Could you check a few things on this drawing? It's one solid part, dimensions in mm from its lowest x, y, z. A direction names the side the tool comes from. Give positions to 0.01 mm unless a question says otherwise; leave off trailing zeros. Loops run counter-clockwise (first coordinate to the right, second up) from the corner with the lowest first, then second, coordinate; pieces in that order, holes last.
Q1. Suppose I cut it at A-A (x = 25). List the corners of the cut face in (y, z) for me.
Q2. Thinking about a two-plate mould opening in Z: for the marked faces 1, 2 and 3, which applies, pulls with the +Z half, pulls with the -Z half, needs draft (parallel to the pull), parting line crosses it, or undercut?
Q3. I'm going to push a flat-ended pin straight in: P1, Ø6, axis at y = 23, z = 22, coming from the +X side. Where does the tip first touch, or does it pass through?
Q4. Suppose I cut it at C-C (y = 30). List the corners of the cut face in (x, z) for me.
Q5. Suppose I cut it at B-B (z = 20). List the corners of the cut face in (x, y) for me.
Q6. I need wall thicknesses on probe 1 along X at (y, z) = (11, 35); probe 2 along Z at (x, y) = (7, 14) (1 decimal); probe 3 along Z at (x, y) = (33, 12.5). Which ranges of each line are inside material? Lowest first, please.
Q7. Suppose I cut it at D-D (z = 24.5). List the corners of the cut face in (x, y) for me, and give its area (3 significant figures).
Q8. For the marked faces 4 and 5, which set-ups out of +Z, -Z, +X, -X, +Y, -Y let a thin tool reach every point of the face, with its end or its side?
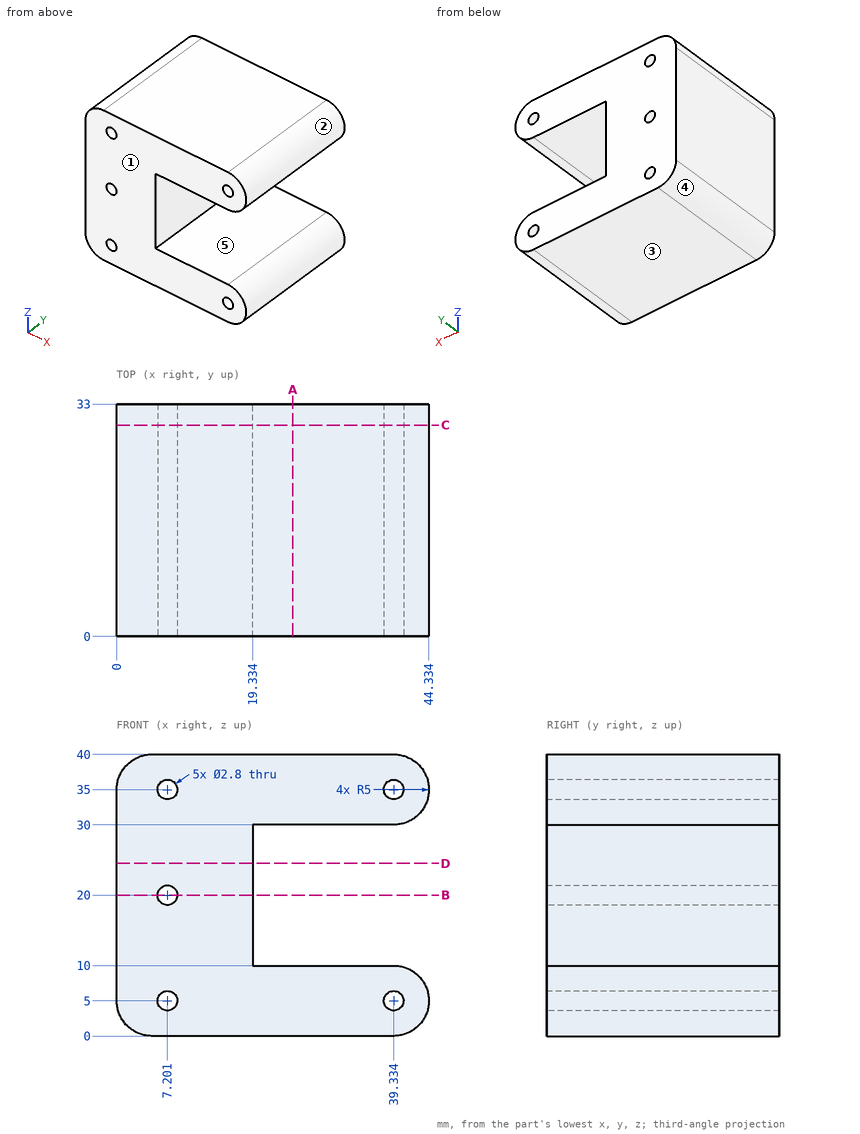
Solutions:
1. outline: (0, 0) - (33, 0) - (33, 10) - (0, 10) - close; (0, 30) - (33, 30) - (33, 40) - (0, 40) - close
2. face 1: needs draft
2. face 2: undercut
2. face 3: pulls with the -Z half
3. P1: stops at x = 19.33
4. outline: (0, 5) arc R5 ccw to (5, 0) - (39.33, 0) arc R5 ccw to (39.33, 10) - (19.33, 10) - (19.33, 30) - (39.33, 30) arc R5 ccw to (39.33, 40) - (5, 40) arc R5 ccw to (0, 35) - close; hole circle Ø2.8 at (7.2, 5); hole circle Ø2.8 at (7.2, 20); hole circle Ø2.8 at (7.2, 35); hole circle Ø2.8 at (39.33, 5); hole circle Ø2.8 at (39.33, 35)
5. outline: (0, 0) - (5.8, 0) - (5.8, 33) - (0, 33) - close; (8.6, 0) - (19.33, 0) - (19.33, 33) - (8.6, 33) - close
6. probe 1: x = 0 to 5.8, 8.6 to 37.93, 40.73 to 44.33
6. probe 2: z = 0 to 3.6, 6.4 to 18.6, 21.4 to 33.6, 36.4 to 40
6. probe 3: z = 0 to 10, 30 to 40
7. outline: (0, 0) - (19.33, 0) - (19.33, 33) - (0, 33) - close
7. area: 638 mm2
8. face 4: -Z, -X, +Y, -Y
8. face 5: +X, +Y, -Y
